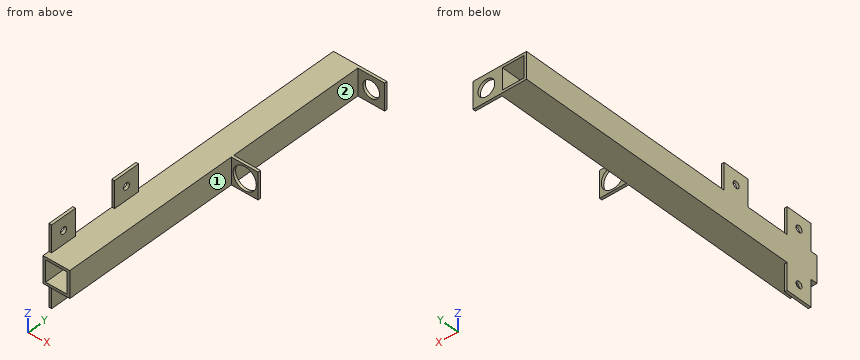
Autodesk Inventor part; units mm, degrees
ref_plane "YZ Plane" through (0, 0, 0) normal (1, 0, 0) x (0, 1, 0)
ref_plane "XZ Plane" through (0, 0, 0) normal (0, 1, 0) x (-1, 0, 0)
ref_plane "XY Plane" through (0, 0, 0) normal (0, 0, 1) x (1, 0, 0)
sketch "Sketch1" plane through (0, 0, 0) normal (0, 1, 0) x (-1, 0, 0)
  line L0 (0, 0) -> (25.4, 0)
  line L1 (25.4, 0) -> (25.4, -25.4)
  line L2 (25.4, -25.4) -> (0, -25.4)
  line L3 (0, -25.4) -> (0, 0)
  dimension "d0" = 25.4
  dimension "d1" = 25.4
extrude "Extrusion1" add sketch "Sketch1" along normal blind 307.975
sketch "Sketch2" plane through (0, 307.975, 0) normal (0, 1, 0) x (1, 0, 0)
  line L0 (-22.86, 2.54) -> (-2.54, 2.54)
  line L1 (-2.54, 2.54) -> (-2.54, 22.86)
  line L2 (-2.54, 22.86) -> (-22.86, 22.86)
  line L3 (-22.86, 22.86) -> (-22.86, 2.54)
  line L4 (-25.4, 0) -> (0, 0)
  line L5 (-25.4, 25.4) -> (-25.4, 0)
  dimension "d4" = 20.32
  dimension "d5" = 20.32
  dimension "d6" = 2.54
  dimension "d7" = 2.54
extrude "Extrusion2" cut sketch "Sketch2" against normal blind 307.975
sketch "Sketch3" plane through (0, 0, 0) normal (1, 0, 0) x (0, 0, -1)
  line L0 (0, 0) -> (0, 307.975)
  line L1 (0, 307.975) -> (25.4, 307.975)
  line L2 (25.4, 307.975) -> (25.4, 305.435)
  line L3 (25.4, 305.435) -> (0, 305.435)
  line L4 (0, 305.435) -> (0, 307.975)
  dimension "d10" = 25.4
  dimension "d11" = 2.54
extrude "Extrusion3" add sketch "Sketch3" along normal blind 25.4
sketch "Sketch4" plane through (0, 307.975, 0) normal (0, 1, 0) x (1, 0, 0)
  circle A0 centre (12.7, 12.7) radius 7.9121
  line L0 (-25.4, 0) -> (25.4, 0)
  line L1 (25.4, 25.4) -> (25.4, 0)
  point P0 (0, 0)
  dimension "d14" = 15.8242
  dimension "d15" = 12.7
  dimension "d16" = 12.7
extrude "Extrusion4" cut sketch "Sketch4" against normal blind 25.4
sketch "Sketch5" plane through (0, 0, 0) normal (1, 0, 0) x (0, 0, -1)
  line L0 (0, 173.8561) -> (25.4, 173.8561)
  line L1 (25.4, 173.8561) -> (25.4, 171.3161)
  line L2 (25.4, 171.3161) -> (0, 171.3161)
  line L3 (0, 171.3161) -> (0, 173.8561)
  point P0 (0, 0)
  dimension "d19" = 25.4
  dimension "d20" = 2.54
extrude "Extrusion5" add sketch "Sketch5" along normal blind 25.4
sketch "Sketch6" plane through (0, 171.3161, -25.4) normal (0, -1, 0) x (1, 0, 0)
  circle A0 centre (12.7, 12.7) radius 10.9601
  line L0 (0, 0) -> (25.4, 0)
  line L1 (25.4, 25.4) -> (25.4, 0)
  point P0 (0, 25.4)
  dimension "d23" = 21.9202
  dimension "d24" = 12.7
  dimension "d25" = 1.7399
extrude "Extrusion6" cut sketch "Sketch6" against normal blind 25.4
sketch "Sketch7" plane through (-25.4, 0, 0) normal (0, 0, 1) x (1, 0, 0)
  line L0 (0, 0) -> (0, 307.975)
  line L1 (0, 31.75) -> (2.54, 31.75)
  line L2 (2.54, 31.75) -> (2.54, 6.35)
  line L3 (2.54, 6.35) -> (0, 6.35)
  line L4 (0, 6.35) -> (0, 31.75)
  line L5 (25.4, 0) -> (0, 0)
  line L6 (0, 0) -> (0, 307.975)
  line L7 (2.54, 307.975) -> (2.54, 0)
  line L8 (0, 73.025) -> (2.54, 73.025)
  line L9 (2.54, 73.025) -> (2.54, 98.425)
  line L10 (2.54, 98.425) -> (0, 98.425)
  line L11 (0, 98.425) -> (0, 73.025)
  dimension "d28" = 2.54
  dimension "d30" = 6.35
  dimension "d48" = 25.4
  dimension "d49" = 25.4
  dimension "d50" = 41.275
sketch "Sketch8" plane through (0, 0, -25.4) normal (0, 0, -1) x (-1, 0, 0)
  line L0 (25.4, 0) -> (25.4, 307.975)
  line L1 (25.4, 31.75) -> (22.86, 31.75)
  line L2 (22.86, 31.75) -> (22.86, 6.35)
  line L3 (22.86, 6.35) -> (25.4, 6.35)
  line L4 (25.4, 6.35) -> (25.4, 31.75)
  line L5 (25.4, 0) -> (0, 0)
  dimension "d33" = 2.54
  dimension "d34" = 25.4
  dimension "d35" = 31.75
extrude "Extrusion8" add sketch "Sketch8" along normal blind 25.4
sketch "Sketch10" plane through (-22.86, 6.35, -25.4) normal (1, 0, 0) x (0, 0, -1)
  circle A0 centre (12.7, 12.7) radius 3.175
  line L0 (0, 0) -> (25.4, 0)
  line L1 (0, -6.35) -> (0, 164.9661)
  point P0 (-25.4, -6.35)
  dimension "d43" = 6.35
  dimension "d44" = 12.7
  dimension "d45" = 12.7
extrude "Extrusion10" cut sketch "Sketch10" against normal blind 25.4
extrude "Extrusion11" add sketch "Sketch7" along normal blind 25.4 contours L0 L1 L2 L3 | L0 L10 L7 L8
sketch "Sketch11" plane through (-22.86, 73.025, 0) normal (1, 0, 0) x (0, 0, -1)
  circle A0 centre (-12.7, -53.975) radius 3.175
  line L0 (0, -41.275) -> (-25.4, -41.275)
  line L1 (-12.7, -41.275) -> (-12.7, -53.975) construction
  line L2 (-12.7, -53.975) -> (-25.4, -53.975) construction
  circle A1 centre (-12.7, 12.7) radius 3.175
  line L3 (-12.7, 12.7) -> (-12.7, 25.4) construction
  line L4 (0, 25.4) -> (-25.4, 25.4)
  line L5 (-12.7, 12.7) -> (-25.4, 12.7) construction
  point P0 (0, -73.025)
  dimension "d53" = 6.35
  dimension "d54" = 12.7
  dimension "d55" = 6.35
  dimension "d56" = 12.7
extrude "Extrusion12" cut sketch "Sketch11" against normal blind 25.4
properties part number "Mount for Control Panel"
The model under review builds one solid part; all positions refer to its coordinate system, in mm. Face numbers are marked on the shaded views. Round coordinates to 2 decimals unless told otherwise and drop trailing zeros. Order: outer loops, then holes, each group sorted by start corner. A loop starts at its lowest first (then second) coordinate and runs counter-clockwise, first axis right, second up. Notation, with made-up numbers: (43, 17) -> (77, 17) arc R26 ccw to (77, 39) -> close; hole circle Ø10 at (-30, -25). An arc over 180 degrees is marked (long way). One line per item, written item: value. Start each with the question number.
Q1. Take a section at C-C (x = 12.7). Write out the cut boundary in (y, z) (3 decimals).
Q2. Wall thickness on line 1 (Y direction, x = -24.6, z = 12.7) (3 decimals); line 2 (Z direction, x = 12.7, y = 306.5); line 3 (X direction, y = 289, z = -9): over which ranges is each line inside the solid? List them lowest first.
Q3. Clearance check with flat-ended pins moving along their axes: pin 1 Ø14 at (x, z) = (12.7, -12.7) entering from -Y; pin 2 Ø16.5 at (y, z) = (131, -12) entering from +X; pin 3 Ø3 at (x, z) = (-23.5, -41) entering from -Y; pin 4 Ø10 at (x, y) = (-11.5, 215.5) entering from +Z. State where each tip first meets the part, or that it passes through.
Q4. Take a section at B-B (x = -5.5). Write out the cut boundary in (y, z) (3 decimals), and give its area (3 significant figures).
Q5. Take a section at A-A (y = 19.05). Write out the cut boundary in (x, z) (3 decimals).
Q6. Take a section at D-D (z = -12.7). Write out the cut boundary in (x, y) (3 decimals), and give its area (3 significant figures).
Q7. Mouldability with a two-part tool opening along Y and no side actions: class the marked faces 1 and 2 as released by +Y, released by -Y, zero draft, split by the parting line, or undercut.
Reported:
1. outline: (171.316, -25.4) -> (173.856, -25.4) -> (173.856, -23.66) -> (171.316, -23.66) -> close; (171.316, -1.74) -> (173.856, -1.74) -> (173.856, 0) -> (171.316, 0) -> close; (305.435, -25.4) -> (307.975, -25.4) -> (307.975, -20.612) -> (305.435, -20.612) -> close; (305.435, -4.788) -> (307.975, -4.788) -> (307.975, 0) -> (305.435, 0) -> close
2. line 1: y = 6.35 to 15.875, 22.225 to 31.75, 73.025 to 82.55, 88.9 to 98.425
2. line 2: z = -25.4 to -20.61, -4.79 to 0
2. line 3: x = -25.4 to -22.86, -2.54 to 0
3. pin 1: passes through
3. pin 2: stops at x = 0
3. pin 3: stops at y = 6.35
3. pin 4: stops at z = 0
4. outline: (0, -25.4) -> (307.975, -25.4) -> (307.975, -22.86) -> (0, -22.86) -> close; (0, -2.54) -> (307.975, -2.54) -> (307.975, 0) -> (0, 0) -> close
4. area: 1,560 mm2
5. outline: (-25.4, -50.8) -> (-22.86, -50.8) -> (-22.86, -41.275) -> (-25.4, -41.275) -> close; (-25.4, -34.925) -> (-22.86, -34.925) -> (-22.86, -25.4) -> (0, -25.4) -> (0, 0) -> (-22.86, 0) -> (-22.86, 9.525) -> (-25.4, 9.525) -> close; (-25.4, 15.875) -> (-22.86, 15.875) -> (-22.86, 25.4) -> (-25.4, 25.4) -> close; hole (-22.86, -22.86) -> (-2.54, -22.86) -> (-2.54, -2.54) -> (-22.86, -2.54) -> close
6. outline: (-25.4, 0) -> (-22.86, 0) -> (-22.86, 307.975) -> (-25.4, 307.975) -> close; (-2.54, 0) -> (0, 0) -> (0, 171.316) -> (1.74, 171.316) -> (1.74, 173.856) -> (0, 173.856) -> (0, 305.435) -> (4.788, 305.435) -> (4.788, 307.975) -> (-2.54, 307.975) -> close; (20.612, 305.435) -> (25.4, 305.435) -> (25.4, 307.975) -> (20.612, 307.975) -> close; (23.66, 171.316) -> (25.4, 171.316) -> (25.4, 173.856) -> (23.66, 173.856) -> close
6. area: 1,600 mm2
7. face 1: zero draft
7. face 2: undercut
